Geometry check sheet. Reference: the model listing, model coordinates, mm. Face numbers are marked on the shaded views. A direction names the side the tool comes from. Give positions to 0.01 mm unless a question says otherwise; leave off trailing zeros. Order: outer loops, then holes, each group sorted by start corner. A loop starts at its lowest first (then second) coordinate and runs counter-clockwise, first axis right, second up. Notation, with made-up numbers: M 48.25,-18 L 102.25,-18 A32 cw 102.25,13 Z; hole C 36.5,-2.75 d9. An arc over 180 degrees is marked long. One line per question, with ' | ' between items. Start each with the question number.
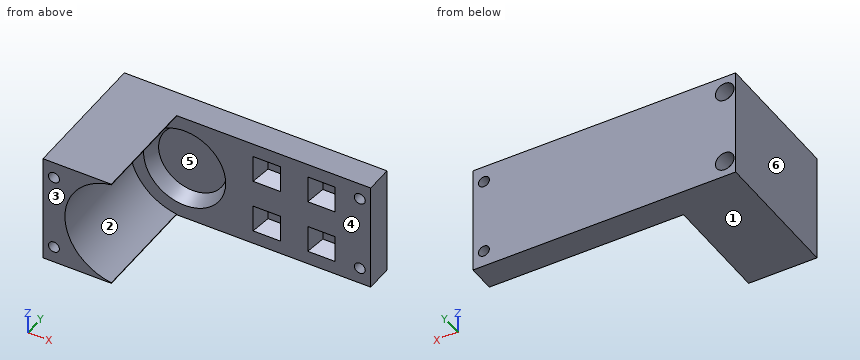
Autodesk Fusion 360 part; units mm, degrees
sketch "baseplate" plane through (0, 0, 0) normal (0, 1, 0) x (1, 0, 0)
  line L0 (0, 0) -> (80, 0)
  line L1 (80, 0) -> (80, -40)
  line L2 (80, -40) -> (0, -40)
  line L3 (0, -40) -> (0, 0)
  dimension "d1" = 40
  dimension "d2" = 80
extrude "Extrude1" add sketch "baseplate" along normal blind 10
sketch "outside_pryamid" plane through (0, 0, 0) normal (0, 1, 0) x (1, 0, 0)
  line L0 (45, -35) -> (55, -35)
  line L1 (55, -35) -> (55, -25)
  line L2 (55, -25) -> (45, -25)
  line L3 (45, -25) -> (45, -35)
  line L4 (65, -35) -> (75, -35)
  line L5 (75, -35) -> (75, -25)
  line L6 (75, -25) -> (65, -25)
  line L7 (65, -25) -> (65, -35)
  line L8 (45, -15) -> (55, -15)
  line L9 (55, -15) -> (55, -5)
  line L10 (55, -5) -> (45, -5)
  line L11 (45, -5) -> (45, -15)
  line L12 (65, -15) -> (75, -15)
  line L13 (75, -15) -> (75, -5)
  line L14 (75, -5) -> (65, -5)
  line L15 (65, -5) -> (65, -15)
  circle A0 centre (20, -20) radius 15
  dimension "d40" = 30
ref_plane "WorkPlane1" through (0, 5, 0) normal (0, 1, 0) x (0, 0, 1)
sketch "inside_pryamid" plane through (0, 5, 0) normal (0, 1, 0) x (1, 0, 0)
  line L0 (47.5, -7.5) -> (47.5, -10)
  line L1 (47.5, -12.5) -> (52.5, -12.5)
  line L2 (52.5, -7.5) -> (47.5, -7.5)
  line L3 (47.5, -10) -> (47.5, -12.5)
  line L4 (52.5, -12.5) -> (52.5, -7.5)
  line L5 (67.5, -10) -> (67.5, -12.5)
  line L6 (67.5, -12.5) -> (72.5, -12.5)
  line L7 (67.5, -7.5) -> (67.5, -10)
  line L8 (72.5, -12.5) -> (72.5, -7.5)
  line L9 (72.5, -7.5) -> (67.5, -7.5)
  line L10 (67.5, -10) -> (67.5, -12.5)
  line L11 (67.5, -12.5) -> (72.5, -12.5)
  line L12 (72.5, -12.5) -> (72.5, -7.5)
  line L13 (47.5, -7.5) -> (47.5, -10)
  line L14 (52.5, -12.5) -> (52.5, -7.5)
  line L15 (72.5, -7.5) -> (67.5, -7.5)
  line L16 (47.5, -10) -> (47.5, -12.5)
  line L17 (52.5, -7.5) -> (47.5, -7.5)
  line L18 (67.5, -7.5) -> (67.5, -10)
  line L19 (47.5, -12.5) -> (52.5, -12.5)
  line L20 (72.5, -32.5) -> (72.5, -27.5)
  line L21 (72.5, -27.5) -> (67.5, -27.5)
  line L22 (67.5, -30) -> (67.5, -32.5)
  line L23 (72.5, -27.5) -> (67.5, -27.5)
  line L24 (67.5, -27.5) -> (67.5, -30)
  line L25 (47.5, -30) -> (47.5, -32.5)
  line L26 (67.5, -27.5) -> (67.5, -30)
  line L27 (67.5, -30) -> (67.5, -32.5)
  line L28 (67.5, -32.5) -> (72.5, -32.5)
  line L29 (72.5, -32.5) -> (72.5, -27.5)
  line L30 (47.5, -32.5) -> (52.5, -32.5)
  line L31 (47.5, -32.5) -> (52.5, -32.5)
  line L32 (67.5, -32.5) -> (72.5, -32.5)
  line L33 (52.5, -32.5) -> (52.5, -27.5)
  line L34 (52.5, -27.5) -> (47.5, -27.5)
  line L35 (52.5, -27.5) -> (47.5, -27.5)
  line L36 (47.5, -30) -> (47.5, -32.5)
  line L37 (52.5, -32.5) -> (52.5, -27.5)
  line L38 (47.5, -27.5) -> (47.5, -30)
  line L39 (47.5, -27.5) -> (47.5, -30)
  circle A0 centre (20, -20) radius 12.5
  dimension "d42" = 25
loft "Loft9" cut profiles "inside_pryamid", "outside_pryamid" section 1 contours A0 section 2 contours A0
loft "Loft3" cut profiles "outside_pryamid", "inside_pryamid" section 1 contours L0 L1 L2 L3 section 2 contours L25 L30 L31 L33 L34 L35 L36 L37 L38 L39
loft "Loft4" cut profiles "inside_pryamid", "outside_pryamid" section 1 contours L20 L21 L22 L23 L24 L26 L27 L28 L29 L32 section 2 contours L4 L5 L6 L7
loft "Loft7" cut profiles "inside_pryamid", "outside_pryamid" section 1 contours L0 L1 L2 L3 L4 L13 L14 L16 L17 L19 section 2 contours L8 L9 L10 L11
loft "Loft8" cut profiles "inside_pryamid", "outside_pryamid" section 1 contours L5 L6 L7 L8 L9 L10 L11 L12 L15 L18 section 2 contours L12 L13 L14 L15
sketch "sidewall" plane through (0, 0, 0) normal (0, 1, 0) x (1, 0, 0)
  line L0 (-8, 0) -> (-8, -40)
  circle A0 centre (20, -20) radius 20
  line L1 (17, -20) -> (17, -40)
  line L2 (-8, -40) -> (17, -40)
  line L3 (17, -20) -> (17, 0)
  line L4 (-8, 0) -> (17, 0)
  dimension "d43" = 20
  dimension "d44" = 20
extrude "Extrude2" add sketch "sidewall" along normal blind -40 and the other way blind -10 contours L0 A0 L1 L2 L3 L4
sketch "sidemount" plane through (0, 0, 0) normal (0, 1, 0) x (1, 0, 0)
  line L0 (80, 0) -> (88, 0)
  line L1 (88, 0) -> (88, -40)
  line L2 (88, -40) -> (80, -40)
  line L3 (80, -40) -> (80, 0)
extrude "Extrude3" add sketch "sidemount" along normal blind 10
sketch "holes" plane through (0, 0, 0) normal (0, 1, 0) x (1, 0, 0)
  circle A0 centre (-4, -34) radius 2
  circle A1 centre (-4, -6) radius 2
  circle A2 centre (-4, -34) radius 3.4
  circle A3 centre (-4, -6) radius 3.4
  line L0 (88, 0) -> (84, 0)
  line L1 (84, 0) -> (84, -6)
  line L2 (84, -6) -> (88, -6)
  line L3 (88, -6) -> (88, 0)
  circle A4 centre (84, -34) radius 2
  circle A5 centre (84, -6) radius 2
  dimension "d19" = 4
  dimension "d20" = 4
  dimension "d21" = 6.8
  dimension "d22" = 6.8
  dimension "d25" = 4
  dimension "d26" = 6
  dimension "d27" = 4
  dimension "d28" = 4
extrude "Extrude4" cut sketch "holes" against normal blind 50 contours A0 | A1
extrude "Extrude5" cut sketch "holes" along normal blind 40 contours L1 L2 A5 | L1 L2 A5 | A4
extrude "Extrude6" cut sketch "holes" along normal through all and the other way blind 44 contours A0 | A1
extrude "Extrude7" cut sketch "holes" along normal blind 10 and the other way blind -4 contours A2 | A3
Item 1: Cross-section at B-B, the plane x = 20. Record the cut outline in (y, z).
Item 2: Cross-section at C-C, the plane y = -16. Record the cut outline in (x, z), plus the area to 3 significant figures.
Item 3: Cross-section at D-D, the plane x = 84. Record the cut outline in (y, z), plus the area to 3 significant figures.
Item 4: Mould release check, pull along Z, two halves, no side actions. Record for the marked faces 1, 2 and 3: released by +Z, released by -Z, zero draft, split by the parting line, or undercut.
Item 5: Set-up check for the marked faces 4, 5 and 6: record each of +Z, -Z, +X, -X, +Y, -Y from which the full face is reachable in a straight line by a thin tool's end or side.
Item 6: Depth check by flat-ended pin: pin 1 (1.5 mm diameter, centred on x = 70.5, z = 29, fed in from -Y); pin 2 (20 mm diameter, centred on x = 33.5, z = 20.5, fed in from -Y); pin 3 (9 mm diameter, centred on x = -4, z = 34, fed in from +Y); pin 4 (5.5 mm diameter, centred on x = 69.5, z = 10.5, fed in from -Y). Enter the tip coordinate at first touch or a pass-through.
Item 7: Material ranges on line 1 along X through (y, z) = (5.75, 6); line 2 along Z through (x, y) = (-4, -20); line 3 along X through (y, z) = (3.75, 34), recorded low to high.
Item 8: Cross-section at A-A, the plane x = -4. Record the cut outline in (y, z), plus the area to 3 significant figures.
Outcome:
1) outline: M 0,0 L 10,0 L 10,40 L 0,40 L 0,35 L 5,32.5 L 5,7.5 L 0,5 Z
2) outline: M -8,0 L 17,0 L 17,0.23 A20 cw 17,39.77 L 17,40 L -8,40 Z; hole C -4,6 d4; hole C -4,34 d4 | area: 466 mm²
3) outline: M 0,0 L 10,0 L 10,4 L 0,4 Z; M 0,8 L 10,8 L 10,32 L 0,32 Z; M 0,36 L 10,36 L 10,40 L 0,40 Z | area: 320 mm²
4) face 1: released by -Z | face 2: undercut | face 3: zero draft
5) face 4: +X, -Y | face 5: -Y | face 6: +Z, -Z, -X, +Y, -Y
6) pin 1: stops at y = 5 | pin 2: stops at y = 0 | pin 3: stops at y = 10 | pin 4: stops at y = 3.5
7) line 1: x = -8 to -7.4, -0.6 to 82, 86 to 88 | line 2: z = 0 to 4, 8 to 32, 36 to 40 | line 3: x = -8 to -6, -2 to 82, 86 to 88
8) outline: M -40,0 L 10,0 L 10,2.6 L 4,2.6 L 4,4 L -40,4 Z; M -40,8 L 4,8 L 4,9.4 L 10,9.4 L 10,30.6 L 4,30.6 L 4,32 L -40,32 Z; M -40,36 L 4,36 L 4,37.4 L 10,37.4 L 10,40 L -40,40 Z | area: 1,570 mm²
